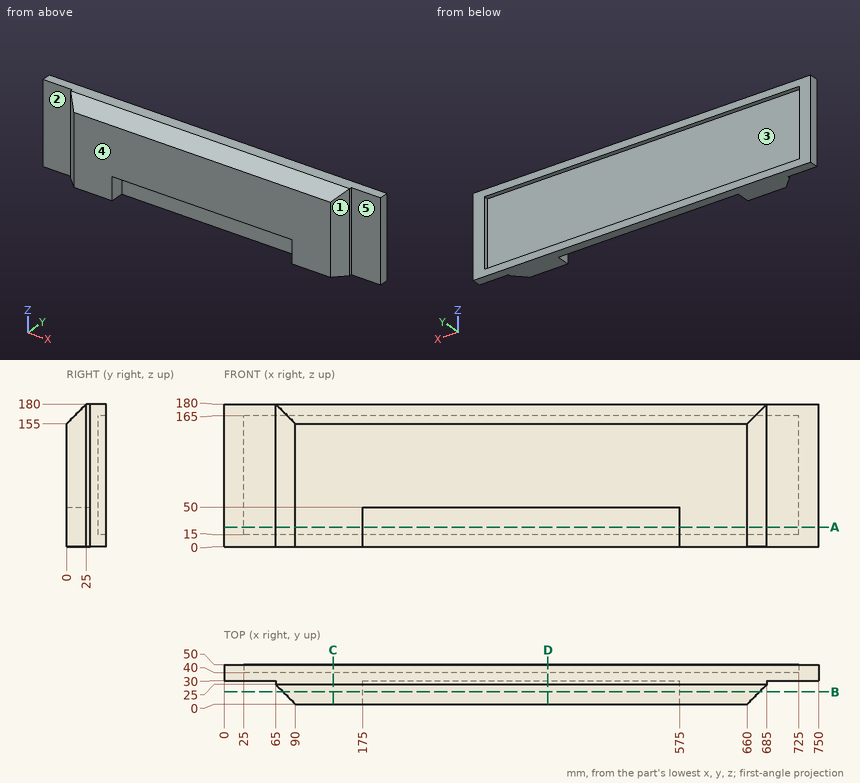
Geometry: see drawing. Coordinates: mm, zero at the bounding-box minimum. A direction names the side the tool comes from. Give positions to 0.01 mm unless a question says otherwise; leave off trailing zeros. Order: outer loops, then holes, each group sorted by start corner. A loop starts at its lowest first (then second) coordinate and runs counter-clockwise, first axis right, second up. Notation, with made-up numbers: M 9.5,-22 L 39.5,-22 A27 ccw 39.5,14 Z; hole C 68,-19.5 d6. An arc over 180 degrees is marked long. Answer as CSV lines item,"result". Start each with the question number.
1) Cut plane C-C (x = 137.5). Output: boundary loops of the cut face in (y, z).
2) Set-up query: the marked faces 4 and 5. Return all of +Z, -Z, +X, -X, +Y, -Y with unobstructed straight access to the full face (end or side cutting, diameter ignored); none if empty.
3) Cut plane A-A (z = 24.5). Output: boundary loops of the cut face in (x, y), then the cut area to 3 significant figures.
4) First-contact query: P1, Ø8, axis at y = 41, z = 141.5, coming from the -X side; P2, Ø4, axis at y = 27.5, z = 79.5, coming from the -X side; P3, Ø6, axis at x = 489.5, y = 13, coming from the +Z side; P4, Ø4, axis at y = 20.5, z = 29, coming from the +X side. Flat tips, straight axial feed; report the tip coordinate or a pass-through.
5) Cut plane D-D (x = 408.5). Output: boundary loops of the cut face in (y, z), then the cut area to 3 significant figures.
6) Mould query, pull axis X, two halves, no side actions, for the marked faces 1, 2 and 3. Classes: +X half, -X half, draft (parallel to the pull), parting line (faces both ways), or undercut.
7) Line query: line 1 (Z direction, x = 63, y = 45); line 2 (X direction, y = 42, z = 38.5); line 3 (Y direction, x = 598, z = 84.5). Output: solid intervals per line, ascending. Write a range as from..to.
8) Cut plane B-B (y = 15.5). Output: boundary loops of the cut face in (x, z), then the cut area to 3 significant figures.
Findings below:
1,outline,"M 0,0 L 50,0 L 50,15 L 40,15 L 40,165 L 50,165 L 50,180 L 25,180 L 0,155 Z"
2,face 4,"+Z, -Z, +X, -X, -Y"
2,face 5,"+Z, -Z, +X, -Y"
3,outline,"M 0,30 L 65,30 L 65,25 L 90,0 L 175,0 L 175,30 L 575,30 L 575,0 L 660,0 L 685,25 L 685,30 L 750,30 L 750,50 L 725,50 L 725,40 L 25,40 L 25,50 L 0,50 Z"
3,area,"14,000 mm²"
4,P1,"stops at x = 0"
4,P2,"stops at x = 65"
4,P3,"stops at z = 171"
4,P4,"stops at x = 682.5"
5,outline,"M 0,50 L 30,50 L 30,0 L 50,0 L 50,15 L 40,15 L 40,165 L 50,165 L 50,180 L 25,180 L 0,155 Z"
5,area,"5,690 mm²"
6,face 1,"+X half"
6,face 2,"draft"
6,face 3,"undercut"
7,line 1,"z = 0..15, 165..180"
7,line 2,"x = 0..25, 725..750"
7,line 3,"y = 0..40"
8,outline,"M 74.5,0 L 175,0 L 175,50 L 575,50 L 575,0 L 675.5,0 L 675.5,170.5 L 74.5,170.5 Z"
8,area,"82,500 mm²"
